Geometry check sheet. Reference: the model listing, model coordinates, mm. A direction names the side the tool comes from. Coordinates: 2 decimals unless noted, no trailing zeros. Loops run counter-clockwise (first coordinate to the right, second up) from the corner with the lowest first, then second, coordinate; pieces in that order, holes last. Notation, with made-up numbers: (-32.5, 53) -> (-9.5, 53) arc R33 ccw to (-9.5, 81) -> close; hole circle Ø2 at (78, -9). An arc over 180 degrees is marked (long way). Answer as a JSON object with one key per item and string values.
from build123d import *

# Parameters (mm, degrees)
F0_R     = 21
F1_DEPTH = 200
F4_R     = 20
F4_R_2   = 17
F5_DEPTH = 25


with BuildPart() as f1:
    # F0 (on Top) → F1 (new body)
    with BuildSketch(Plane.XY):
        Circle(F0_R)
    extrude(amount=F1_DEPTH)

    # F2 (on Front) → F3 (revolve)
    with BuildSketch(Plane.XZ):
        Polygon((-24, 185), (0, 185), (0, 241), (-24, 241), (-29, 236), (-29, 218), (-24, 213), align=None)
    revolve(axis=Axis((0, 0, 74.559175), (0, 0, 1)))

    # F4 (on face) → F5 (join)
    with BuildSketch(Plane.XY.offset(241)):
        Circle(F4_R)
        Circle(F4_R_2, mode=Mode.SUBTRACT)
    extrude(amount=F5_DEPTH)


solid = f1.part
1. Thickness scan on probe 1 along Y at (x, z) = (0, 257); probe 2 along Z at (x, y) = (-2.5, 14); probe 3 along Y at (x, z) = (-3.5, 255.5). Record the ranges inside material, lowest first. Write a range as from..to.
Evaluation:
{"probe 1": "y = -20..-17, 17..20", "probe 2": "z = 0..241", "probe 3": "y = -19.69..-16.64, 16.64..19.69"}
2. Mould release check, pull along X, two halves, no side actions. Record for faces 1 (the face through (0.1, 21.2, 185)), 2 (the face through (0, 0, 241)), 3 (the face through (-4.336, -19.524, 253.325)): released by +X, released by -X, zero draft, split by the parting line, or undercut.
Evaluation:
{"face 1": "zero draft", "face 2": "undercut", "face 3": "split by the parting line"}
3. Section check D-D, the plane z = 203. Record the boundary of the cut face in (x, y), then the cut area to 3 significant figures.
Evaluation:
{"outline": "circle Ø48 at (0, 0)", "area": "1,810 mm^2"}
4. Section check C-C, the plane z = 249.5. Record the boundary of the cut face in (x, y).
Evaluation:
{"outline": "circle Ø40 at (0, 0); hole circle Ø34 at (0, 0)"}
5. Depth check by flat-ended pin: P1, Ø10, axis at x = 7.5, y = -5, coming from the +Z side; P2, Ø2, axis at y = 7, z = 123, coming from the -X side; P3, Ø3, axis at y = -16.5, z = 154.5, coming from the +X side. Enter the tip coordinate at first touch or a pass-through.
Evaluation:
{"P1": "stops at z = 241", "P2": "stops at x = -20.12", "P3": "stops at x = 14.7"}
6. Tool access check on faces 4 (the face through (0, 0, 0)), 5 (the face through (9.139, 14.334, 253.325)), 6 (the face through (23.977, -1.055, 198.804)). Record the directions out of +Z, -Z, +X, -X, +Y, -Y that give a thin tool (end or side, any length) a straight path to the whole face; none if there is none.
Evaluation:
{"face 4": "-Z, +X, -X, +Y, -Y", "face 5": "+Z", "face 6": "-Z"}
7. Section check A-A, the plane y = 0. Record the boundary of the cut face in (x, z), then the cut area to 3 significant figures.
Evaluation:
{"outline": "(-29, 218) -> (-24, 213) -> (-24, 185) -> (-21, 185) -> (-21, 0) -> (21, 0) -> (21, 185) -> (24, 185) -> (24, 213) -> (29, 218) -> (29, 236) -> (24, 241) -> (20, 241) -> (20, 266) -> (17, 266) -> (17, 241) -> (-17, 241) -> (-17, 266) -> (-20, 266) -> (-20, 241) -> (-24, 241) -> (-29, 236) -> close", "area": "10,800 mm^2"}
